Answer from the drawing. Dimensions are ordinates in mm from the lowest x, y and z of the part. Coordinates: 2 decimals unless noted, no trailing zeros. Loops run counter-clockwise (first coordinate to the right, second up) from the corner with the lowest first, then second, coordinate; pieces in that order, holes last. Notation, with made-up numbers: (46, 64.5) - (99, 64.5) arc R16 cw to (99, 68.5) - close; hole circle Ø7 at (57.5, 32.5). An arc over 180 degrees is marked (long way). Use one line per item in the form item = value. Start each with the question number.
1) A cutting plane is placed at D-D (z = 54). Give the vertices of the cut face in (x, y) (1 decimal).
2) Each of these flat-tipped pins is pushed along its axis until it touches: P1, Ø2, axis at x = 20.5, y = 46.5, coming from the -Z side; P2, Ø3, axis at x = 21, z = 67, coming from the -Y side (1 decimal); P3, Ø10, axis at x = 38.5, z = 55, coming from the -Y side (1 decimal); P4, Ø10, axis at x = 16.5, y = 88.5, coming from the +Z side (1 decimal). Where does it stop, or does it pass through?
3) A cutting plane is placed at C-C (y = 90). Give the vertices of the cut face in (x, z).
4) A cutting plane is placed at A-A (y = 77). Give the vertices of the cut face in (x, z), and give its area (3 significant figures).
5) The mould has two halves that part along Z. Classify the marked faces 1, 2, 3 and 4: released by +Z, released by -Z, zero draft, split by the parting line, or undercut.
6) Consider line 1 (Z direction, x = 31.5, y = 26.5) (1 decimal); line 2 (Z direction, x = 48, y = 29.5) (1 decimal); line 3 (Y direction, x = 28, z = 68.5). Determine where each line is inside the solid, lowest interval first.
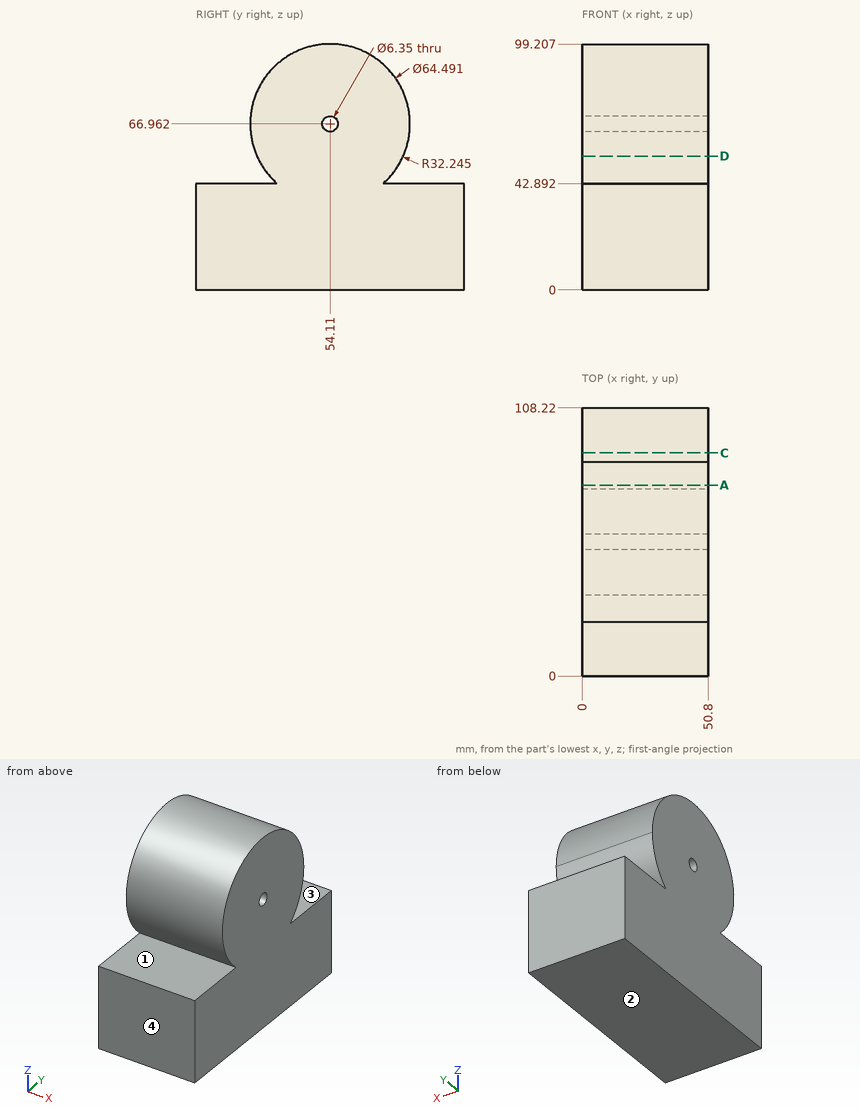
Found:
q1.outline = (0, 24.6) - (50.8, 24.6) - (50.8, 83.6) - (0, 83.6) - close
q2.P1 = 0
q2.P2 = 21.9
q2.P3 = 22.6
q2.P4 = 80.2
q3.outline = (0, 0) - (50.8, 0) - (50.8, 42.89) - (0, 42.89) - close
q4.outline = (0, 0) - (50.8, 0) - (50.8, 42.89) - (0, 42.89) - close; (0, 44.25) - (50.8, 44.25) - (50.8, 89.67) - (0, 89.67) - close
q4.area = 4,490 mm^2
q5.face_1 = undercut
q5.face_2 = released by -Z
q5.face_3 = undercut
q5.face_4 = zero draft
q6.line_1 = 0 to 42.9, 50.3 to 83.6
q6.line_2 = 0 to 42.9, 46.1 to 87.8
q6.line_3 = 21.9 to 51.33, 56.89 to 86.32
